The listing builds one solid part. Answer for the finished solid, in the listing's coordinates (mm). A direction names the side the tool comes from. Coordinates: 2 decimals unless noted, no trailing zeros. Order: outer loops, then holes, each group sorted by start corner. A loop starts at its lowest first (then second) coordinate and runs counter-clockwise, first axis right, second up. Notation, with made-up numbers: (55, -3.5) -> (67, -3.5) arc R27 cw to (67, 27.5) -> close; hole circle Ø9 at (3, 53.5). An arc over 180 degrees is marked (long way). Return JSON: item names as keys, results as strings.
```python
from build123d import *

# Parameters (mm, degrees)
ESQUISSE1_W        = 20
ESQUISSE1_H        = 20
ESQUISSE1_R        = 2
BOSS_EXTRU_1_DEPTH = 4
ESQUISSE2_W        = 20
ESQUISSE2_H        = 20
BOSS_EXTRU_2_DEPTH = 4
BOSS_EXTRU_3_DEPTH = 4
BOSS_EXTRU_4_DEPTH = 4
ESQUISSE5_W        = 4.5
ESQUISSE5_H        = 4
BOSS_EXTRU_5_DEPTH = 3
CONG_1_R           = 3
CONG_2_R           = 2


with BuildPart() as part:
    # Esquisse1 → Boss.-Extru.1 (new body)
    with BuildSketch(Plane.XY):
        Rectangle(ESQUISSE1_W, ESQUISSE1_H)
        with Locations((0, -4)):
            Circle(ESQUISSE1_R, mode=Mode.SUBTRACT)
    extrude(amount=BOSS_EXTRU_1_DEPTH)

    # Esquisse2 → Boss.-Extru.2 (add)
    with BuildSketch(Plane(origin=(0, 10, 0), x_dir=(1, 0, 0), z_dir=(0, 1, 0))):
        with Locations((0, -10)):
            Rectangle(ESQUISSE2_W, ESQUISSE2_H)
    extrude(amount=-BOSS_EXTRU_2_DEPTH)

    # Esquisse3 → Boss.-Extru.3 (add)
    with BuildSketch(Plane.ZY.offset(10)):
        Polygon((4, -10), (20, 6), (4, 6), align=None)
    extrude(amount=-BOSS_EXTRU_3_DEPTH)

    # Esquisse4 → Boss.-Extru.4 (add)
    with BuildSketch(Plane(origin=(10, 0, 0), x_dir=(0, 0, -1), z_dir=(1, 0, 0))):
        Polygon((-20, 6), (-4, 6), (-4, -10), align=None)
    extrude(amount=-BOSS_EXTRU_4_DEPTH)

    # Esquisse5 → Boss.-Extru.5 (add)
    with BuildSketch(Plane(origin=(0, 0, 0), x_dir=(-1, 0, 0), z_dir=(0, 0, -1))):
        with Locations((0, 8)):
            Rectangle(ESQUISSE5_W, ESQUISSE5_H)
    extrude(amount=BOSS_EXTRU_5_DEPTH)

    # Congé1
    cong_1_edges = [part.edges().sort_by_distance(p)[0] for p in [
        (6.125, 10, 0),
        (10, 0, 0),
        (-10, 0, 0),
        (-6.125, 10, 0),
        (-10, 10, 10),
        (10, 10, 10),
    ]]
    fillet(cong_1_edges, radius=CONG_1_R)

    # Congé2
    cong_2_edges = [part.edges().sort_by_distance(p)[0] for p in [
        (-2.25, 10, 0),
    ]]
    fillet(cong_2_edges, radius=CONG_2_R)
    cong_2_2_edges = [part.edges().sort_by_distance(p)[0] for p in [
        (1, 10, -3),
    ]]
    fillet(cong_2_2_edges, radius=CONG_2_R)
    cong_2_3_edges = [part.edges().sort_by_distance(p)[0] for p in [
        (2.25, 10, 1),
    ]]
    fillet(cong_2_3_edges, radius=CONG_2_R)
    cong_2_4_edges = [part.edges().sort_by_distance(p)[0] for p in [
        (-2.25, 6, -0.5),
    ]]
    fillet(cong_2_4_edges, radius=CONG_2_R - 0.0001)  # a hair under: the kernel refuses the full size


solid = part.part
```
Item 1: Find the intervals of material crossed by probe 1 along Y at (x, z) = (0, 2.6); probe 2 along X at (y, z) = (-5.5, 5.5); probe 3 along Z at (x, y) = (2.25, 0.5), in increasing order.
Answer list:
{"probe 1": "-10 to -6, -2 to 10", "probe 2": "-10 to -6, 6 to 10", "probe 3": "0 to 4"}
Item 2: The part is cut by section B-B on x = 5.25. Determine the outline of the cut face in (y, z).
Answer list:
{"outline": "(-10, 0) -> (7, 0) arc R3 ccw to (10, 3) -> (10, 20) -> (6, 20) -> (6, 4) -> (-10, 4) -> close"}
Item 3: The part is cut by section A-A on y = -4. Determine the outline of the cut face in (x, z), plus the area to 3 significant figures.
Answer list:
{"outline": "(-10, 3) arc R3 ccw to (-7, 0) -> (-2, 0) -> (-2, 4) -> (-6, 4) -> (-6, 10) -> (-10, 10) -> close; (2, 0) -> (7, 0) arc R3 ccw to (10, 3) -> (10, 10) -> (6, 10) -> (6, 4) -> (2, 4) -> close", "area": "108 mm2"}
Item 4: The part is cut by section C-C on z = 9.75. Determine the outline of the cut face in (x, y).
Answer list:
{"outline": "(-10, -4.25) -> (-6, -4.25) -> (-6, 6) -> (6, 6) -> (6, -4.25) -> (10, -4.25) -> (10, 7) arc R3 ccw to (7, 10) -> (-7, 10) arc R3 ccw to (-10, 7) -> close"}
Item 5: Flat-ended cylindrical pins translate along their axes: pin 1 (1.5 mm diameter, centred on y = -7.5, z = 2, fed in from +X); pin 2 (11 mm diameter, centred on x = 1.5, y = 0, fed in from -Z); pin 3 (5 mm diameter, centred on x = 0, y = -4, fed in from +Z). Find the tip coordinate at first contact, or state that the pin passes through.
Answer list:
{"pin 1": "x = 9.99", "pin 2": "z = 0", "pin 3": "z = 4"}
Item 6: Determine the mould class of faces 1 (the flat face through (6, 0, 10)), 2 (the flat face through (0, 6, 12)), 3 (the cylindrical face through (4.42, 9.1, 0.86)), 4 (the flat face through (-10, 1, 9)) for opening direction X: pulls with the +X half, pulls with the -X half, needs draft (parallel to the pull), parting line crosses it, or undercut.
Answer list:
{"face 1": "undercut", "face 2": "undercut", "face 3": "needs draft", "face 4": "pulls with the -X half"}
Item 7: Which of the six approach directions +Z, -Z, +X, -X, +Y, -Y give full straight-line access (tool end or side, diameter ignored) to faces 5 (the cylindrical face through (-9.14, -1.62, 0.9)), 6 (the flat face through (-1, -2, 4))?
Answer list:
{"face 5": "-Z, -X, +Y, -Y", "face 6": "+Z, -Y"}
Item 8: The part is cut by section D-D on y = -0.75. Determine the outline of the cut face in (x, z), plus the area to 3 significant figures.
Answer list:
{"outline": "(-10, 3) arc R3 ccw to (-7, 0) -> (7, 0) arc R3 ccw to (10, 3) -> (10, 13.25) -> (6, 13.25) -> (6, 4) -> (-6, 4) -> (-6, 13.25) -> (-10, 13.25) -> close", "area": "150 mm2"}
